Build history of the part. All positions in model axes, mm. Round coordinates to 2 decimals unless told otherwise and drop trailing zeros. Write each loop counter-clockwise with the first axis right and the second up, starting at its lowest first coordinate (ties: lowest second). Pieces come first, ordered by that corner, then holes.
Item 1: Band-saw the part on B-B, the plane z = 3. Write the cut outline in (x, y), then the cut area to 3 significant figures.
Item 2: Band-saw the part on C-C, the plane y = -109.5. Write the cut outline in (x, z), then the cut area to 3 significant figures.
Item 3: Wall check: probe 1 along Y at (x, z) = (2.5, 7.75); probe 2 along X at (y, z) = (-89.5, 6.75); probe 3 along X at (y, z) = (-85, 7.25). Give the ranges that are in metal, low to high.
Item 4: Band-saw the part on A-A, the plane y = -82. Write the cut outline in (x, z), then the cut area to 3 significant figures.
Item 5: Drop a flat-ended pin along its axis: pin 1 Ø10 at (x, y) = (47.5, -71) entering from +Z. Give the stop position or say it passes through.
Item 6: Band-saw the part on D-D, the plane x = -27. Write the cut outline in (y, z), then the cut area to 3 significant figures.
```python
from build123d import *

# Parameters (mm, degrees)
EXTRUDE1_DEPTH = 8


with BuildPart() as part:
    # Sketch1 → Extrude1 (new body)
    with BuildSketch(Plane.XY):
        with BuildLine():
            Line((-103.894448725, 0), (103.894448725, 0))
            ThreePointArc((103.894448725, 0), (105.310022501, -0.354976204), (106.390599608, -1.335899411))
            Line((106.390599608, -1.335899411), (114.996150883, -14.244226325))
            ThreePointArc((114.996150883, -14.244226325), (115.371276079, -15.038974467), (115.5, -15.908326913))
            Line((115.5, -15.908326913), (115.5, -122))
            ThreePointArc((115.5, -122), (114.621320344, -124.121320344), (112.5, -125))
            Line((112.5, -125), (104.871428571, -125))
            ThreePointArc((104.871428571, -125), (103.624149291, -124.728423427), (102.602691232, -123.96286293))
            Line((102.602691232, -123.96286293), (56.718433491, -70.928426739))
            ThreePointArc((56.718433491, -70.928426739), (0, -45), (-56.718433491, -70.928426739))
            Line((-56.718433491, -70.928426739), (-102.602691232, -123.96286293))
            ThreePointArc((-102.602691232, -123.96286293), (-103.624149291, -124.728423427), (-104.871428571, -125))
            Line((-104.871428571, -125), (-112.5, -125))
            ThreePointArc((-112.5, -125), (-114.621320344, -124.121320344), (-115.5, -122))
            Line((-115.5, -122), (-115.5, -15.908326913))
            ThreePointArc((-115.5, -15.908326913), (-115.371276079, -15.038974467), (-114.996150883, -14.244226325))
            Line((-114.996150883, -14.244226325), (-106.390599608, -1.335899411))
            ThreePointArc((-106.390599608, -1.335899411), (-105.310022501, -0.354976204), (-103.894448725, 0))
        make_face()
    extrude(amount=EXTRUDE1_DEPTH)


solid = part.part
```
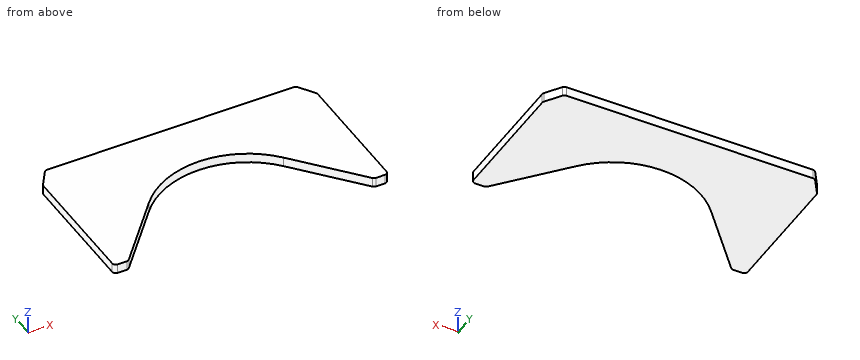
Results:
1. outline: (-115.5, -122) arc R3 ccw to (-112.5, -125) - (-104.87, -125) arc R3 ccw to (-102.6, -123.96) - (-56.72, -70.93) arc R75 cw to (56.72, -70.93) - (102.6, -123.96) arc R3 ccw to (104.87, -125) - (112.5, -125) arc R3 ccw to (115.5, -122) - (115.5, -15.91) arc R3 ccw to (115, -14.24) - (106.39, -1.34) arc R3 ccw to (103.89, 0) - (-103.89, 0) arc R3 ccw to (-106.39, -1.34) - (-115, -14.24) arc R3 ccw to (-115.5, -15.91) - close
1. area: 18,000 mm2
2. outline: (-115.5, 0) - (-90.09, 0) - (-90.09, 8) - (-115.5, 8) - close; (90.09, 0) - (115.5, 0) - (115.5, 8) - (90.09, 8) - close
2. area: 407 mm2
3. probe 1: y = -45.04 to 0
3. probe 2: x = -115.5 to -72.79, 72.79 to 115.5
3. probe 3: x = -115.5 to -68.89, 68.89 to 115.5
4. outline: (-115.5, 0) - (-66.3, 0) - (-66.3, 8) - (-115.5, 8) - close; (66.3, 0) - (115.5, 0) - (115.5, 8) - (66.3, 8) - close
4. area: 787 mm2
5. pin 1: passes through
6. outline: (-50.03, 0) - (0, 0) - (0, 8) - (-50.03, 8) - close
6. area: 400 mm2
